Job drawing, mm, ordinate dimensions from the low corner. One solid piece. A direction names the side the tool comes from. Round coordinates to 2 decimals unless told otherwise and drop trailing zeros. Loops run counter-clockwise (first coordinate to the right, second up) from the corner with the lowest first, then second, coordinate; pieces in that order, holes last.
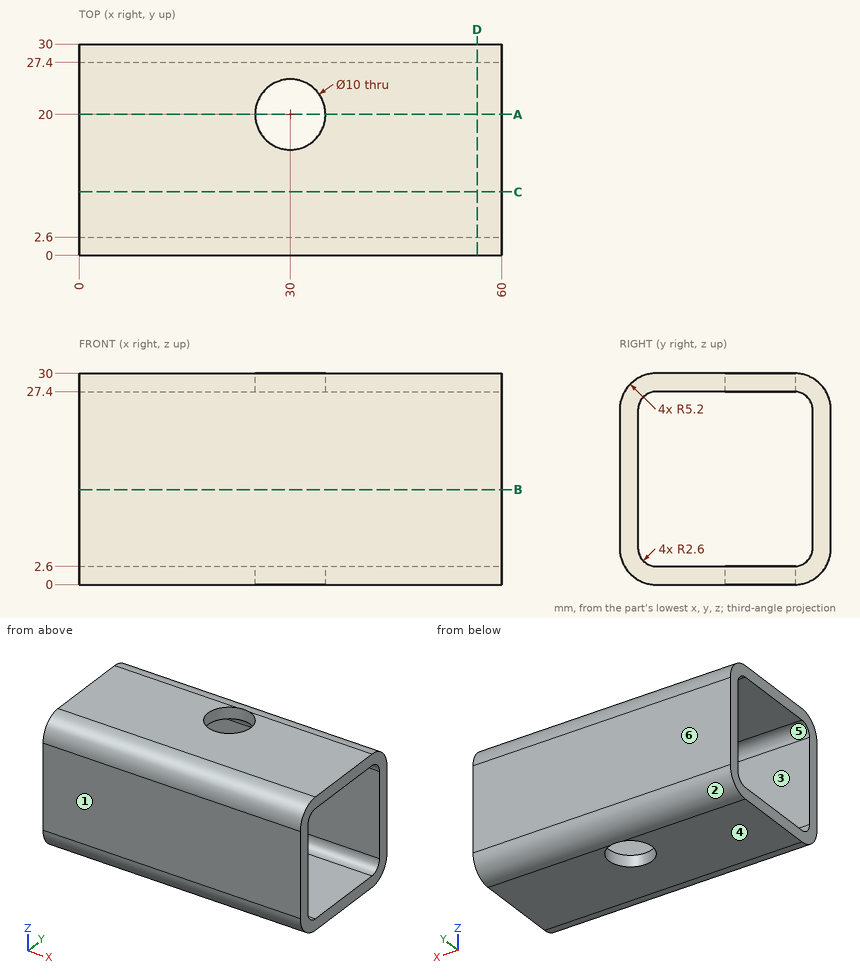
1) Slice it at A-A, the plane y = 20. Give the cut face in (x, z), then the cut area to 3 significant figures.
Values:
outline: (0, 0) - (25, 0) - (25, 2.6) - (0, 2.6) - close; (0, 27.4) - (25, 27.4) - (25, 30) - (0, 30) - close; (35, 0) - (60, 0) - (60, 2.6) - (35, 2.6) - close; (35, 27.4) - (60, 27.4) - (60, 30) - (35, 30) - close
area: 260 mm2
2) Slice it at B-B, the plane z = 13.5. Give the cut face in (x, y), then the cut area to 3 significant figures.
Values:
outline: (0, 0) - (60, 0) - (60, 2.6) - (0, 2.6) - close; (0, 27.4) - (60, 27.4) - (60, 30) - (0, 30) - close
area: 312 mm2
3) Drop a flat-ended pin along its axis: pin 1 Ø10 at (x, y) = (29, 16.5) entering from +Z. Give the stop position or say it passes through.
Values:
pin 1: stops at z = 30
4) Wall check: line 1 along Y through (x, z) = (47.5, 15); line 2 along X through (y, z) = (20, 1). Give the ranges that are in metal, low to high.
Values:
line 1: y = 0 to 2.6, 27.4 to 30
line 2: x = 0 to 25, 35 to 60
5) Mould opens along Y. For the marked faces 1, 2, 3 and 4 say: released by +Y, released by -Y, zero draft, split by the parting line, or undercut.
Values:
face 1: released by -Y
face 2: released by +Y
face 3: undercut
face 4: zero draft
6) Slice it at D-D, the plane x = 56.5. Give the cut face in (y, z).
Values:
outline: (0, 5.2) arc R5.2 ccw to (5.2, 0) - (24.8, 0) arc R5.2 ccw to (30, 5.2) - (30, 24.8) arc R5.2 ccw to (24.8, 30) - (5.2, 30) arc R5.2 ccw to (0, 24.8) - close; hole (2.6, 5.2) arc R2.6 ccw to (5.2, 2.6) - (24.8, 2.6) arc R2.6 ccw to (27.4, 5.2) - (27.4, 24.8) arc R2.6 ccw to (24.8, 27.4) - (5.2, 27.4) arc R2.6 ccw to (2.6, 24.8) - close
7) Tool access for the marked faces 5 and 6: list every direction of +Z, -Z, +X, -X, +Y, -Y with a clear straight run to the whole face (end or side of a thin tool).
Values:
face 5: +X, -X
face 6: +Z, -Z, +X, -X, +Y
